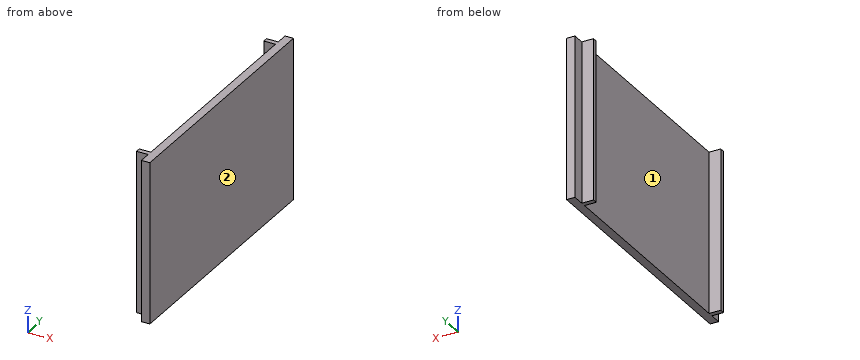
Autodesk Inventor part; units mm, degrees
ref_plane "YZ Plane" through (0, 0, 0) normal (1, 0, 0) x (0, 1, 0)
ref_plane "XZ Plane" through (0, 0, 0) normal (0, 1, 0) x (-1, 0, 0)
ref_plane "XY Plane" through (0, 0, 0) normal (0, 0, 1) x (1, 0, 0)
sketch "Sketch1" plane through (0, 0, 0) normal (0, 0, 1) x (1, 0, 0)
  line L0 (-49.56, 19.825) -> (-47.46, 19.825)
  line L1 (-47.46, 19.825) -> (-47.46, -35.175)
  line L2 (-47.46, -35.175) -> (-49.56, -35.175)
  line L3 (-49.56, -35.175) -> (-49.56, 19.825)
  point P0 (0, 0)
  dimension "d0" = 2.1
  dimension "d1" = 55
extrude "Extrusion1" add sketch "Sketch1" along normal blind 40
sketch "Sketch2" plane through (-47.46, -35.175, 0) normal (1, 0, 0) x (0, 0, -1)
  line L0 (-40, 55) -> (0, 55)
  line L1 (0, 55) -> (0, 56.2)
  line L2 (0, 56.2) -> (-40, 56.2)
  line L3 (-40, 56.2) -> (-40, 55)
  line L4 (0, 0) -> (-40, 0)
  line L5 (-40, 0) -> (-40, -1.2)
  line L6 (-40, -1.2) -> (0, -1.2)
  line L7 (0, -1.2) -> (0, 0)
  line L8 (0, 55) -> (0, 0)
  line L9 (-40, 0) -> (-40, 55)
  point P0 (0, 35.175)
  dimension "d4" = 1.2
  dimension "d5" = 1.2
extrude "Extrusion2" add sketch "Sketch2" against normal blind 5 contours L3 L2 L1 L0 | L4 L7 L6 L5
sketch "Sketch3" plane through (-47.46, 21.025, 40) normal (0, 1, 0) x (1, 0, 0)
  line L0 (0, 40) -> (-2.1, 40)
  line L1 (-2.1, 40) -> (-2.1, 0)
  line L2 (-2.1, 0) -> (0, 0)
  line L3 (0, 0) -> (0, 40)
  point P0 (47.46, 40)
extrude "Extrusion3" add sketch "Sketch3" along normal blind 3
sketch "Sketch4" plane through (-47.46, -36.375, 0) normal (0, -1, 0) x (1, 0, 0)
  line L0 (0, 40) -> (-2.1, 40)
  line L1 (-2.1, 40) -> (-2.1, 0)
  line L2 (-2.1, 0) -> (0, 0)
  line L3 (0, 0) -> (0, 40)
  point P0 (47.46, 0)
extrude "Extrusion4" add sketch "Sketch4" along normal blind 3
properties part number "40mm Side v1"
Here's how the part is built. I have some questions about the finished solid (model axes, mm). Face numbers are marked on the shaded views. Give positions to 0.01 mm unless a question says otherwise; leave off trailing zeros. Loops run counter-clockwise (first coordinate to the right, second up) from the corner with the lowest first, then second, coordinate; pieces in that order, holes last. Notation, with made-up numbers: M 56.25,66 L 93.25,66 A30 cw 93.25,96 Z; hole C 87,53 d5. An arc over 180 degrees is marked long. Put each result on its own line as item: value. Start each with the question number.
(1) If we mould it in two halves opening along Y, with no side actions, what happens to the marked faces 1 and 2? For each: +Y half, -Y half, draft (parallel to the pull), parting line (faces both ways), or undercut.
(2) I need wall thicknesses on line 1 along Y through (x, z) = (-51.85, 34) (3 decimals); line 2 along X through (y, z) = (-19, 33.5). Which ranges of each line are inside material? Lowest first, please. Write a range as [from, to].
(3) I want a section at B-B on z = 14. Please give me the cut outline in (x, y) (3 decimals), then the cut area to 3 significant figures.
(4) Will these pins go through, and if not, where does the flat tip stop? pin 1 Ø1 at (x, y) = (-52, -17) entering from +Z; pin 2 Ø1.4 at (x, z) = (-51, 28.5) entering from +Y (3 decimals); pin 3 Ø3 at (x, z) = (-51.5, 22.5) entering from -Y (3 decimals); pin 4 Ø5 at (y, z) = (-32, 28.5) entering from -X.
(5) I want a section at A-A on x = -51. Please give me the cut outline in (y, z) (3 decimals), then the cut area to 3 significant figures.
(6) I want a section at C-C on y = 4.5. Please give me the cut outline in (x, z), then the cut area to 3 significant figures.
Answer block:
1. face 1: undercut
1. face 2: draft
2. line 1: [-36.375, -35.175], [19.825, 21.025]
2. line 2: [-49.56, -47.46]
3. outline: M -52.46,-36.375 L -49.56,-36.375 L -49.56,-39.375 L -47.46,-39.375 L -47.46,24.025 L -49.56,24.025 L -49.56,21.025 L -52.46,21.025 L -52.46,19.825 L -49.56,19.825 L -49.56,-35.175 L -52.46,-35.175 Z
3. area: 140 mm^2
4. pin 1: through
4. pin 2: y = 21.025
4. pin 3: y = -36.375
4. pin 4: x = -49.56
5. outline: M -36.375,0 L -35.175,0 L -35.175,40 L -36.375,40 Z; M 19.825,0 L 21.025,0 L 21.025,40 L 19.825,40 Z
5. area: 96.0 mm^2
6. outline: M -49.56,0 L -47.46,0 L -47.46,40 L -49.56,40 Z
6. area: 84.0 mm^2
